Job drawing, mm, ordinate dimensions from the low corner. One solid piece. Give positions to 0.01 mm unless a question says otherwise; leave off trailing zeros. Loops run counter-clockwise (first coordinate to the right, second up) from the corner with the lowest first, then second, coordinate; pieces in that order, holes last. Notation, with made-up numbers: (4.5, 67.25) -> (25.5, 67.25) arc R25 cw to (25.5, 85.25) -> close; hole circle Ø11 at (65.5, 47.25). An arc over 180 degrees is marked (long way). Use one line per item in the form item = value.
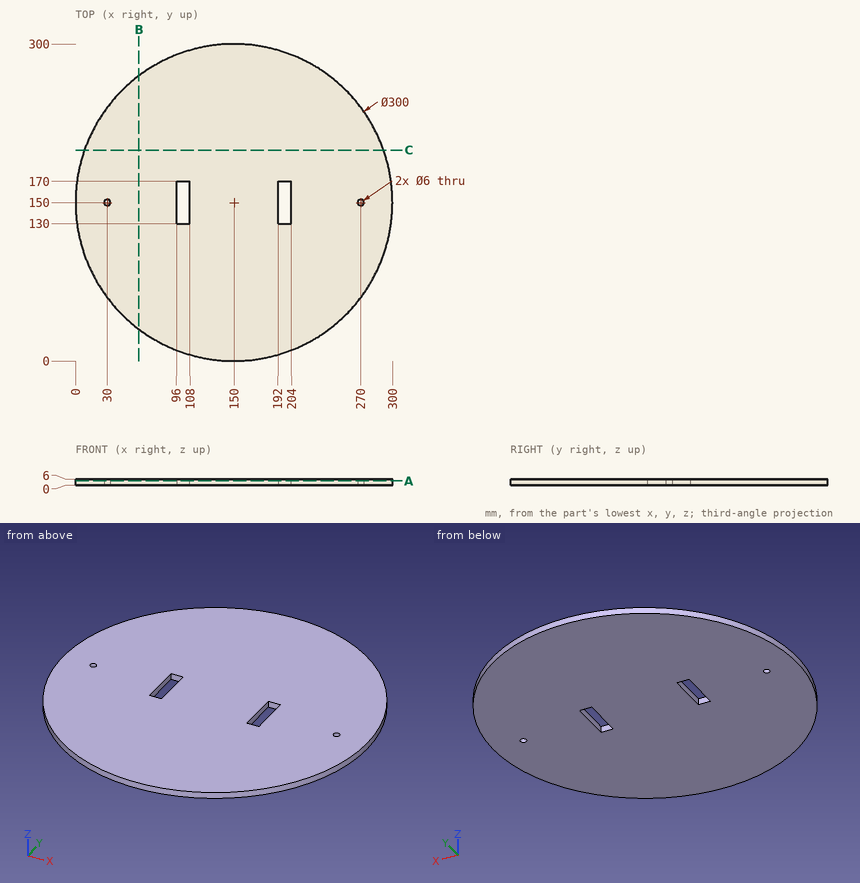
1. Drill centre lines: line 1 (X direction, y = 157, z = 0.2); line 2 (X direction, y = 166.5, z = 3.3); line 3 (X direction, y = 151, z = 1.9). Where is each one in solid material? Low to high.
Result sheet:
line_1 = 0.16 to 96, 108 to 192, 204 to 299.84
line_2 = 0.91 to 96, 108 to 192, 204 to 299.09
line_3 = 0 to 27.17, 32.83 to 96, 108 to 192, 204 to 267.17, 272.83 to 300
2. Cut at C-C, the plane y = 199.5. Write the cut outline in (x, z), then the cut area to 3 significant figures.
Result sheet:
outline = (8.4, 0) -> (291.6, 0) -> (291.6, 6) -> (8.4, 6) -> close
area = 1,700 mm^2
3. Cut at B-B, the plane x = 60. Write the cut outline in (y, z), then the cut area to 3 significant figures.
Result sheet:
outline = (30, 0) -> (270, 0) -> (270, 6) -> (30, 6) -> close
area = 1,440 mm^2
4. Cut at A-A, the plane z = 4.2. Write the cut outline in (x, y), then the cut area to 3 significant figures.
Result sheet:
outline = circle Ø300 at (150, 150); hole circle Ø6 at (30, 150); hole (96, 130) -> (108, 130) -> (108, 170) -> (96, 170) -> close; hole (192, 130) -> (204, 130) -> (204, 170) -> (192, 170) -> close; hole circle Ø6 at (270, 150)
area = 69,700 mm^2
5. Drop flat-ended pins along their axis: P1, Ø1.8, axis at y = 155.5, z = 3.5, coming from the +X side; P2, Ø3, axis at x = 99.5, z = 2.5, coming from the +Y side; P3, Ø5.5, axis at x = 30, y = 150, coming from the +Z side; P4, Ø1.5, axis at y = 64, z = 4.5, coming from the +X side. Give the stop position or say it passes through.
Result sheet:
P1 = 299.93
P2 = 291.77
P3 = through
P4 = 273.42
